Design review of the part built by this model. Coordinates are the model's own, in mm. A direction names the side the tool comes from. Coordinates: 2 decimals unless noted, no trailing zeros. Write each loop counter-clockwise with the first axis right and the second up, starting at its lowest first coordinate (ties: lowest second). Pieces come first, ordered by that corner, then holes. Notation, with made-up numbers: (50.5, 14) - (69.5, 14) arc R15 cw to (69.5, 35) - close; hole circle Ø3 at (11.25, -3.5). An arc over 180 degrees is marked (long way). Answer as a JSON object with one key per item and string values.
```python
from build123d import *

# Parameters (mm, degrees)
SKETCH1_W           = 93.85
SKETCH1_H           = 63.5
SKETCH1_R           = 1.65
BOSS_EXTRUDE1_DEPTH = 1.6
FILLET1_R           = 4
SKETCH2_W           = 53.5
SKETCH2_H           = 26.3
BOSS_EXTRUDE2_DEPTH = 3.8
SKETCH3_W           = 9.3
SKETCH3_H           = 7.8
BOSS_EXTRUDE3_DEPTH = 4
SKETCH4_W           = 9.7
SKETCH4_H           = 8.6
SKETCH4_W_2         = 6.151959396
BOSS_EXTRUDE4_DEPTH = 4.9


with BuildPart() as part:
    # Sketch1 → Boss-Extrude1 (new body)
    with BuildSketch(Plane(origin=(0, 0, 0), x_dir=(1, 0, 0), z_dir=(0, 1, 0))):
        Rectangle(SKETCH1_W, SKETCH1_H)
        with Locations((-43.1625, 27.95)):
            Circle(SKETCH1_R, mode=Mode.SUBTRACT)
        with Locations((43.1625, 27.95)):
            Circle(SKETCH1_R, mode=Mode.SUBTRACT)
        with Locations((43.1625, -27.95)):
            Circle(SKETCH1_R, mode=Mode.SUBTRACT)
        with Locations((-43.1625, -27.95)):
            Circle(SKETCH1_R, mode=Mode.SUBTRACT)
    extrude(amount=BOSS_EXTRUDE1_DEPTH)

    # Fillet1
    fillet1_edges = [part.edges().sort_by_distance(p)[0] for p in [
        (46.925, 0.8, 31.75),
        (-46.925, 0.8, 31.75),
        (-46.925, 0.8, -31.75),
        (46.925, 0.8, -31.75),
    ]]
    fillet(fillet1_edges, radius=FILLET1_R)

    # Sketch2 → Boss-Extrude2 (add)
    with BuildSketch(Plane(origin=(0, 1.6, 0), x_dir=(1, 0, 0), z_dir=(0, 1, 0))):
        with Locations((13.075, 0)):
            Rectangle(SKETCH2_W, SKETCH2_H)
    extrude(amount=BOSS_EXTRUDE2_DEPTH)

    # Sketch3 → Boss-Extrude3 (add)
    with BuildSketch(Plane(origin=(0, 5.4, 0), x_dir=(1, 0, 0), z_dir=(0, 1, 0))):
        with Locations((37.175, 0)):
            Rectangle(SKETCH3_W, SKETCH3_H)
    extrude(amount=BOSS_EXTRUDE3_DEPTH)

    # Sketch4 → Boss-Extrude4 (add)
    with BuildSketch(Plane(origin=(0, 1.6, 0), x_dir=(1, 0, 0), z_dir=(0, 1, 0))):
        with Locations((7.775, -17.45)):
            Rectangle(SKETCH4_W, SKETCH4_H)
        with Locations((-20.075, -17.45)):
            Rectangle(SKETCH4_W, SKETCH4_H)
        with Locations((-30.200979698, -17.45)):
            Rectangle(SKETCH4_W_2, SKETCH4_H)
    extrude(amount=BOSS_EXTRUDE4_DEPTH)


solid = part.part
```
(1) Take a section at B-B, the plane x = -23. Write out the cut boundary in (y, z), and give its area (3 significant figures).
Solved:
{"outline": "(0, -31.75) - (1.6, -31.75) - (1.6, 13.15) - (6.5, 13.15) - (6.5, 21.75) - (1.6, 21.75) - (1.6, 31.75) - (0, 31.75) - close", "area": "144 mm^2"}
(2) The part is to be moulded in two halves that separate along X. For faces 4 (the face through (2.925, 4, 18)), 5 (the face through (-30, 4, 13.15)), 6 (the face through (39.825, 3, 0)), say which applies: pulls with the +X half, pulls with the -X half, needs draft (parallel to the pull), parting line crosses it, or undercut.
Solved:
{"face 4": "undercut", "face 5": "needs draft", "face 6": "pulls with the +X half"}
(3) Take a section at C-C, the plane z = 11. Write out the cut boundary in (x, y) (3 decimals).
Solved:
{"outline": "(-46.925, 0) - (46.925, 0) - (46.925, 1.6) - (39.825, 1.6) - (39.825, 5.4) - (-13.675, 5.4) - (-13.675, 1.6) - (-46.925, 1.6) - close"}
(4) For pin 1 (4.5 mm diameter, centred on x = 35.5, y = 7.5, fed in from -Z); pin 2 (1.5 mm diameter, centred on y = 5, z = 17, fed in from +X) (3 decimals); pin 3 (3 mm diameter, centred on y = 4.5, z = -2, fed in from +X) (3 decimals); pin 4 (4 mm diameter, centred on x = -8.5, y = 2.5, fed in from +Z), all flat-tipped, find the tip position at first contact; note any pin that passes through.
Solved:
{"pin 1": "stops at z = -13.15", "pin 2": "stops at x = 12.625", "pin 3": "stops at x = 41.825", "pin 4": "stops at z = 31.75"}
(5) Tool access review of faces 1 (the face through (-13.675, 3, 0)), 2 (the face through (37, 7, 3.9)), 3 (the face through (12.625, 4, 18)): name each direction out of +Z, -Z, +X, -X, +Y, -Y from which nothing blocks a thin tool from reaching the whole face with its end or side.
Solved:
{"face 1": "+Z, -Z, -X, +Y", "face 2": "+Z, +X, -X, +Y", "face 3": "+Z, +X, +Y"}
(6) Take a section at D-D, the plane x = 38.5. Write out the cut boundary in (y, z).
Solved:
{"outline": "(0, -31.75) - (1.6, -31.75) - (1.6, -13.15) - (5.4, -13.15) - (5.4, -3.9) - (9.4, -3.9) - (9.4, 3.9) - (5.4, 3.9) - (5.4, 13.15) - (1.6, 13.15) - (1.6, 31.75) - (0, 31.75) - close"}
(7) To check wall thickness, follow line 1 (X direction, y = 2.5, z = 14) (3 decimals); line 2 (X direction, y = 0.9, z = -27.95); line 3 (Y direction, x = -23, z = 7). State the ranges of each line that lie inside material, in increasing order. Write a range as from..to.
Solved:
{"line 1": "x = -33.277..-27.125, -24.925..-15.225, 2.925..12.625", "line 2": "x = -46.92..-44.81, -41.51..41.51, 44.81..46.92", "line 3": "y = 0..1.6"}
(8) Take a section at A-A, the plane y = 3. Write out the cut boundary in (x, z) (3 decimals), and give its area (3 significant figures).
Solved:
{"outline": "(-33.277, 13.15) - (-27.125, 13.15) - (-27.125, 21.75) - (-33.277, 21.75) - close; (-24.925, 13.15) - (-15.225, 13.15) - (-15.225, 21.75) - (-24.925, 21.75) - close; (-13.675, -13.15) - (39.825, -13.15) - (39.825, 13.15) - (12.625, 13.15) - (12.625, 21.75) - (2.925, 21.75) - (2.925, 13.15) - (-13.675, 13.15) - close", "area": "1,630 mm^2"}
